Source: CAD feature listing. Evaluate the final solid. Frame: model axes, mm. Face numbers are marked on the shaded views. A direction names the side the tool comes from. Round coordinates to 2 decimals unless told otherwise and drop trailing zeros. Order: outer loops, then holes, each group sorted by start corner. A loop starts at its lowest first (then second) coordinate and runs counter-clockwise, first axis right, second up. Notation, with made-up numbers: (-2, 54) -> (39, 54) arc R5 ccw to (39, 59) -> close; hole circle Ø1 at (68.5, 61.25). An arc over 180 degrees is marked (long way). Answer as CSV lines item,"result".
from build123d import *

# Parameters (mm, degrees)
F0_W     = 54
F0_H     = 54
F0_R     = 2.75
F1_DEPTH = 8
F2_R     = 16
F2_R_2   = 10
F3_DEPTH = 80
F4_R     = 4.75
F5_DEPTH = 5.4
F6_R     = 10
F7_DEPTH = 25


with BuildPart() as f1:
    # F0 (on Top) → F1 (new body)
    with BuildSketch(Plane.XY):
        Rectangle(F0_W, F0_H)
        with Locations((-15.202796, -15.202796)):
            Circle(F0_R, mode=Mode.SUBTRACT)
        with Locations((15.202796, -15.202796)):
            Circle(F0_R, mode=Mode.SUBTRACT)
        with Locations((-15.202796, 15.202796)):
            Circle(F0_R, mode=Mode.SUBTRACT)
        with Locations((15.202796, 15.202796)):
            Circle(F0_R, mode=Mode.SUBTRACT)
    extrude(amount=F1_DEPTH)

    # F2 (on face) → F3 (join)
    with BuildSketch(Plane(origin=(0, 0, 0), x_dir=(1, 0, 0), z_dir=(0, 0, -1))):
        Circle(F2_R)
        Circle(F2_R_2, mode=Mode.SUBTRACT)
    extrude(amount=F3_DEPTH)

    # F4 (on face) → F5 (cut)
    with BuildSketch(Plane.XY.offset(8)):
        with Locations((-15.202796, 15.202796)):
            Circle(F4_R)
        with Locations((15.202796, 15.202796)):
            Circle(F4_R)
        with Locations((15.202796, -15.202796)):
            Circle(F4_R)
        with Locations((-15.202796, -15.202796)):
            Circle(F4_R)
    extrude(amount=-F5_DEPTH, mode=Mode.SUBTRACT)

    # F6 (on face) → F7 (cut)
    with BuildSketch(Plane.XY.offset(8)):
        Circle(F6_R)
    extrude(amount=-F7_DEPTH, mode=Mode.SUBTRACT)


solid = f1.part
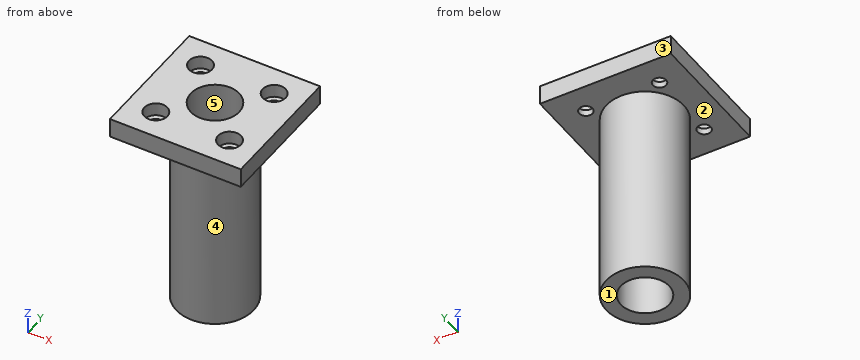
1. Section query D-D on y = 17. Return loops of the section in (x, z), and give its area (3 significant figures).
Results below:
outline,"(-27, 0) -> (-17.28, 0) -> (-17.28, 2.6) -> (-19.6, 2.6) -> (-19.6, 8) -> (-27, 8) -> close; (-13.12, 0) -> (13.12, 0) -> (13.12, 2.6) -> (10.81, 2.6) -> (10.81, 8) -> (-10.81, 8) -> (-10.81, 2.6) -> (-13.12, 2.6) -> close; (17.28, 0) -> (27, 0) -> (27, 8) -> (19.6, 8) -> (19.6, 2.6) -> (17.28, 2.6) -> close"
area,"315 mm2"
2. Line query: L1, parallel to X at y = 0, z = -36; L2, parallel to Z at x = -16.5, y = 25; L3, parallel to Y at x = 4.5, z = -68. Output: solid intervals per line, ascending. Write a range as [from, to].
Results below:
L1,"[-16, -10], [10, 16]"
L2,"[0, 8]"
L3,"[-15.35, -8.93], [8.93, 15.35]"
3. Pin query (flat end, axial travel): pin 1 (6 mm diameter, centred on x = -16, z = -27, fed in from +Y); pin 2 (12 mm diameter, centred on x = 20, y = 6, fed in from -Z); pin 3 (9 mm diameter, centred on x = 15.2, y = -15.2, fed in from -Z); pin 4 (3 mm diameter, centred on x = 17, y = 14, fed in from +Z). Return the tip coordinate at first contact, or that it passes through.
Results below:
pin 1,"y = 9.33"
pin 2,"z = -80"
pin 3,"z = 0"
pin 4,"z = 2.6"
4. Mould query, pull axis X, two halves, no side actions, for the marked faces 3, 4 and 5. Classes: released by +X, released by -X, zero draft, split by the parting line, or undercut.
Results below:
face 3,"zero draft"
face 4,"split by the parting line"
face 5,"undercut"
5. Section query A-A on x = 0. Return loops of the section in (y, z), and give its area (3 significant figures).
Results below:
outline,"(-27, 0) -> (-16, 0) -> (-16, -80) -> (-10, -80) -> (-10, 8) -> (-27, 8) -> close; (10, -80) -> (16, -80) -> (16, 0) -> (27, 0) -> (27, 8) -> (10, 8) -> close"
area,"1,230 mm2"
6. Reachability of the marked faces 1 and 2 from +Z, -Z, +X, -X, +Y, -Y: full face, straight path, thin tool, end or side. Return the list, or none.
Results below:
face 1,"-Z, +X, -X, +Y, -Y"
face 2,"-Z"
7. Section query C-C on z = -57.5. Return loops of the section in (x, y), and give its area (3 significant figures).
Results below:
outline,"circle Ø32 at (0, 0); hole circle Ø20 at (0, 0)"
area,"490 mm2"
